Input: part model. Units: mm. Frame: model coordinates. Round coordinates to 2 decimals unless told otherwise and drop trailing zeros. Loops run counter-clockwise (first coordinate to the right, second up) from the corner with the lowest first, then second, coordinate; pieces in that order, holes last.
1) Section D-D, the plane x = 54.5. Return loops of the section in (y, z).
2) Section C-C, the plane y = 1.3. State how many separate pieces and enclosed holes the cut face has, and give its area (3 significant figures).
3) First-contact query: pin 1 (2 mm diameter, centred on x = -20.86, z = -20.86, fed in from -Y). Flat tip, straight axial feed; report the tip coordinate or a pass-through.
4) Section B-B, the plane x = -63.5. Return loops of the section in (y, z), and give its area (3 significant figures).
5) Section A-A, the plane z = -31.75. Return loops of the section in (x, y), and give its area (3 significant figures).
6) Ray query, line 1 along X through (y, z) = (2.3, -31.75); line 2 along Z through (x, y) = (48, 1.05); line 3 along Z through (x, y) = (20, 4) (3 decimals). Return the intervals inside material, ascending.
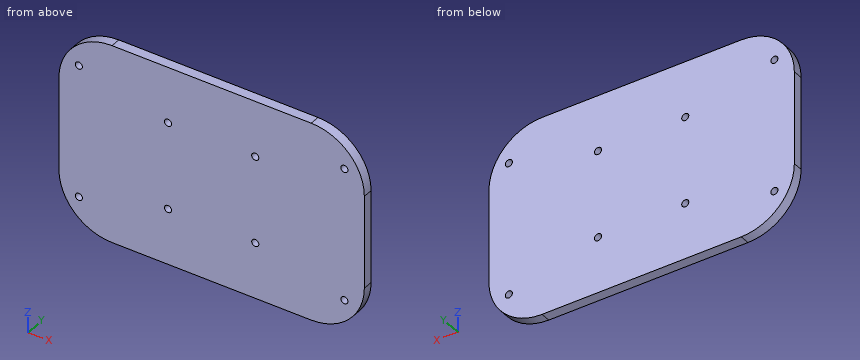
from build123d import *

# Parameters (mm, degrees)
BOSS_EXTRUDE1_DEPTH = 4.7625
SKETCH2_R           = 1.7
CUT_EXTRUDE1_DEPTH  = 88.3125
SKETCH3_R           = 1.7
CUT_EXTRUDE2_DEPTH  = 88.3125


with BuildPart() as part:
    # Sketch1 → Boss-Extrude1 (new body)
    with BuildSketch(Plane(origin=(0, 0, 0), x_dir=(1, 0, 0), z_dir=(0, 1, 0))):
        with BuildLine():
            Line((-47.625, -47.625), (47.625, -47.625))
            ThreePointArc((47.625, -47.625), (65.585512242, -40.185512242), (73.025, -22.225))
            Line((73.025, -22.225), (73.025, 22.225))
            ThreePointArc((73.025, 22.225), (65.585512242, 40.185512242), (47.625, 47.625))
            Line((47.625, 47.625), (-47.625, 47.625))
            ThreePointArc((-47.625, 47.625), (-65.585512242, 40.185512242), (-73.025, 22.225))
            Line((-73.025, 22.225), (-73.025, -22.225))
            ThreePointArc((-73.025, -22.225), (-65.585512242, -40.185512242), (-47.625, -47.625))
        make_face()
    extrude(amount=BOSS_EXTRUDE1_DEPTH)

    # Sketch2 → Cut-Extrude1 (cut, through all)
    with BuildSketch(Plane(origin=(0, 4.7625, 0), x_dir=(1, 0, 0), z_dir=(0, 1, 0))):
        with Locations(Location((-63.5, -31.75, 0), (0, 0, 270))):
            Circle(SKETCH2_R)
        with Locations(Location((-63.5, 31.75, 0), (0, 0, 270))):
            Circle(SKETCH2_R)
        with Locations(Location((63.5, 31.75, 0), (0, 0, 270))):
            Circle(SKETCH2_R)
        with Locations(Location((63.5, -31.75, 0), (0, 0, 270))):
            Circle(SKETCH2_R)
    extrude(amount=-CUT_EXTRUDE1_DEPTH, mode=Mode.SUBTRACT)

    # Sketch3 → Cut-Extrude2 (cut, through all)
    with BuildSketch(Plane(origin=(0, 4.7625, 0), x_dir=(1, 0, 0), z_dir=(0, 1, 0))):
        with Locations(Location((20.859650045, 20.859650045, 0), (0, 0, 270))):
            Circle(SKETCH3_R)
        with Locations(Location((-20.859650045, 20.859650045, 0), (0, 0, 270))):
            Circle(SKETCH3_R)
        with Locations(Location((-20.859650045, -20.859650045, 0), (0, 0, 270))):
            Circle(SKETCH3_R)
        with Locations(Location((20.859650045, -20.859650045, 0), (0, 0, 270))):
            Circle(SKETCH3_R)
    extrude(amount=-CUT_EXTRUDE2_DEPTH, mode=Mode.SUBTRACT)


solid = part.part
Final values:
1. outline: (0, -46.68) - (4.76, -46.68) - (4.76, 46.68) - (0, 46.68) - close
2. separate pieces: 1
2. enclosed holes: 8
2. area: 13,300 mm2
3. pin 1: passes through
4. outline: (0, -42.05) - (4.76, -42.05) - (4.76, -33.45) - (0, -33.45) - close; (0, -30.05) - (4.76, -30.05) - (4.76, 30.05) - (0, 30.05) - close; (0, 33.45) - (4.76, 33.45) - (4.76, 42.05) - (0, 42.05) - close
4. area: 368 mm2
5. outline: (-71.17, 0) - (-65.2, 0) - (-65.2, 4.76) - (-71.17, 4.76) - close; (-61.8, 0) - (61.8, 0) - (61.8, 4.76) - (-61.8, 4.76) - close; (65.2, 0) - (71.17, 0) - (71.17, 4.76) - (65.2, 4.76) - close
5. area: 646 mm2
6. line 1: x = -71.17 to -65.2, -61.8 to 61.8, 65.2 to 71.17
6. line 2: z = -47.62 to 47.62
6. line 3: z = -47.625 to -22.326, -19.393 to 19.393, 22.326 to 47.625
